Part model, mm, in its own coordinate system. Coordinates: 2 decimals unless noted, no trailing zeros. Order: outer loops, then holes, each group sorted by start corner. A loop starts at its lowest first (then second) coordinate and runs counter-clockwise, first axis right, second up. Notation, with made-up numbers: M -18.5,-19 L -5.5,-19 A34 cw -5.5,14 Z; hole C -39,53.5 d1. An arc over 180 degrees is marked long. Write item = value, one per line. Start each with the question number.
Autodesk Inventor part; units mm, degrees
ref_plane "YZ Plane" through (0, 0, 0) normal (1, 0, 0) x (0, 1, 0)
ref_plane "XZ Plane" through (0, 0, 0) normal (0, 1, 0) x (-1, 0, 0)
ref_plane "XY Plane" through (0, 0, 0) normal (0, 0, 1) x (1, 0, 0)
sketch "Sketch1" plane through (0, 0, 0) normal (0, 1, 0) x (-1, 0, 0)
  line L0 (0, 0) -> (53.34, 0)
  line L1 (53.34, 0) -> (53.34, -78.74)
  line L2 (53.34, -78.74) -> (0, -78.74)
  line L3 (0, -78.74) -> (0, 0)
  circle A0 centre (47.3075, -6.35) radius 2.54
  circle A1 centre (47.3075, -60.325) radius 2.54
  circle A2 centre (47.3075, -69.85) radius 2.54
  circle A3 centre (6.0325, -6.35) radius 2.54
  circle A4 centre (6.0325, -60.325) radius 2.54
  circle A5 centre (6.0325, -69.85) radius 2.54
  line L4 (26.67, 0) -> (26.67, -78.74)
  dimension "d0" = 53.34
  dimension "d1" = 78.74
  dimension "d2" = 5.08
  dimension "d3" = 5.08
  dimension "d4" = 5.08
  dimension "d5" = 53.975
  dimension "d6" = 63.5
  dimension "d9" = 41.275
  dimension "d14" = 20.6375
  dimension "d16" = 6.35
extrude "Extrusion1" add sketch "Sketch1" along normal blind 2.54
sketch "Sketch2" plane through (0, 2.54, 0) normal (0, 1, 0) x (1, 0, 0)
  line L0 (-53.34, 0) -> (0, 0)
  line L1 (-53.34, 78.74) -> (-53.34, 0)
  line L2 (0, 78.74) -> (-53.34, 78.74)
  line L3 (0, 0) -> (0, 78.74)
  circle A0 centre (-6.0325, 6.35) radius 2.54
  circle A1 centre (-6.0325, 60.325) radius 2.54
  circle A2 centre (-6.0325, 69.85) radius 2.54
  circle A3 centre (-47.3075, 69.85) radius 2.54
  circle A4 centre (-47.3075, 60.325) radius 2.54
  circle A5 centre (-47.3075, 6.35) radius 2.54
  line L4 (-26.67, 0) -> (-26.67, 78.74)
  line L5 (0, 78.74) -> (-53.34, 78.74)
  line L6 (-26.67, 0) -> (-39.37, 0)
  line L7 (-39.37, 0) -> (-39.37, 78.74)
  line L8 (-39.37, 78.74) -> (-26.67, 78.74)
  line L9 (-26.67, 78.74) -> (-26.67, 0)
  line L10 (-26.67, 0) -> (-13.97, 0)
  line L11 (-13.97, 0) -> (-13.97, 78.74)
  line L12 (-13.97, 78.74) -> (-26.67, 78.74)
  line L13 (-26.67, 78.74) -> (-26.67, 0)
  line L14 (-39.37, 0) -> (-40.386, 0)
  line L15 (-40.386, 0) -> (-40.386, 78.74)
  line L16 (-40.386, 78.74) -> (-39.37, 78.74)
  line L17 (-39.37, 78.74) -> (-39.37, 0)
  line L18 (-26.67, 0) -> (-27.178, 0)
  line L19 (-27.178, 0) -> (-27.178, 78.74)
  line L20 (-27.178, 78.74) -> (-26.67, 78.74)
  line L21 (-26.67, 78.74) -> (-26.67, 0)
  line L22 (-53.34, 0) -> (0, 0)
  line L23 (-26.67, 78.74) -> (-26.162, 78.74)
  line L24 (-26.162, 78.74) -> (-26.162, 0)
  line L25 (-26.162, 0) -> (-26.67, 0)
  line L26 (-26.67, 0) -> (-26.67, 78.74)
  line L27 (-13.97, 0) -> (-12.954, 0)
  line L28 (-12.954, 0) -> (-12.954, 78.74)
  line L29 (-12.954, 78.74) -> (-13.97, 78.74)
  line L30 (-13.97, 78.74) -> (-13.97, 0)
  line L31 (-40.386, 0) -> (-12.954, 0)
  line L32 (-12.954, 0) -> (-12.954, 1.27)
  line L33 (-12.954, 1.27) -> (-40.386, 1.27)
  line L34 (-40.386, 1.27) -> (-40.386, 0)
  line L35 (-12.954, 78.74) -> (-40.386, 78.74)
  line L36 (-40.386, 78.74) -> (-40.386, 77.47)
  line L37 (-40.386, 77.47) -> (-12.954, 77.47)
  line L38 (-12.954, 77.47) -> (-12.954, 78.74)
  line L39 (-53.34, 39.37) -> (0, 39.37)
  line L40 (0, 0) -> (0, 78.74)
  line L41 (-40.386, 39.37) -> (-12.954, 39.37)
  line L42 (-12.954, 39.37) -> (-12.954, 40.005)
  line L43 (-12.954, 40.005) -> (-40.386, 40.005)
  line L44 (-40.386, 40.005) -> (-40.386, 39.37)
  line L45 (-40.386, 39.37) -> (-12.954, 39.37)
  line L46 (-12.954, 39.37) -> (-12.954, 38.735)
  line L47 (-12.954, 38.735) -> (-40.386, 38.735)
  line L48 (-40.386, 38.735) -> (-40.386, 39.37)
  line L49 (-40.386, 38.735) -> (-39.37, 38.735)
  line L50 (-39.37, 38.735) -> (-39.37, 39.37)
  line L51 (-39.37, 39.37) -> (-40.386, 39.37)
  line L52 (-40.386, 39.37) -> (-40.386, 38.735)
  line L53 (-53.34, 78.74) -> (-53.34, 0)
  line L54 (-53.34, 0) -> (-52.324, 0)
  line L55 (-52.324, 0) -> (-52.324, 78.74)
  line L56 (-52.324, 78.74) -> (-53.34, 78.74)
  line L57 (-53.34, 78.74) -> (-53.34, 0)
  line L58 (0, 0) -> (-1.016, 0)
  line L59 (-1.016, 0) -> (-1.016, 78.74)
  line L60 (-1.016, 78.74) -> (0, 78.74)
  line L61 (0, 78.74) -> (0, 0)
  line L62 (-40.386, 39.37) -> (-53.34, 39.37)
  line L63 (-53.34, 39.37) -> (-53.34, 38.735)
  line L64 (-53.34, 38.735) -> (-40.386, 38.735)
  line L65 (-40.386, 38.735) -> (-40.386, 39.37)
  line L66 (-40.386, 39.37) -> (-53.34, 39.37)
  line L67 (-53.34, 39.37) -> (-53.34, 40.005)
  line L68 (-53.34, 40.005) -> (-40.386, 40.005)
  line L69 (-40.386, 40.005) -> (-40.386, 39.37)
  line L70 (-12.954, 39.37) -> (0, 39.37)
  line L71 (0, 39.37) -> (0, 38.735)
  line L72 (0, 38.735) -> (-12.954, 38.735)
  line L73 (-12.954, 38.735) -> (-12.954, 39.37)
  line L74 (-12.954, 39.37) -> (0, 39.37)
  line L75 (0, 39.37) -> (0, 40.005)
  line L76 (0, 40.005) -> (-12.954, 40.005)
  line L77 (-12.954, 40.005) -> (-12.954, 39.37)
  line L78 (-53.34, 38.735) -> (-52.324, 38.735)
  line L79 (-52.324, 38.735) -> (-52.324, 39.37)
  line L80 (-52.324, 39.37) -> (-53.34, 39.37)
  line L81 (-53.34, 39.37) -> (-53.34, 38.735)
  point P0 (-13.97, 38.735)
  point P1 (-13.97, 40.005)
  point P2 (-27.178, 38.735)
  point P3 (-26.162, 38.735)
  point P4 (-26.162, 40.005)
  point P5 (-27.178, 40.005)
  point P6 (-13.97, 1.27)
  point P7 (-27.178, 1.27)
  point P8 (-26.162, 1.27)
  point P9 (-39.37, 1.27)
  point P10 (-13.97, 77.47)
  point P11 (-27.178, 77.47)
  point P12 (-26.162, 77.47)
  point P13 (-39.37, 77.47)
  point P14 (-39.37, 38.735)
  point P15 (-39.37, 40.005)
  point P16 (-1.016, 38.735)
  point P17 (-1.016, 40.005)
  point P18 (-52.324, 38.735)
  point P19 (-52.324, 40.005)
  dimension "d19" = 12.7
  dimension "d20" = 12.7
  dimension "d22" = 0.508
  dimension "d23" = 0.508
  dimension "d24" = 1.016
  dimension "d25" = 1.016
  dimension "d26" = 1.27
  dimension "d27" = 1.27
  dimension "d28" = 0.635
  dimension "d29" = 0.635
  dimension "d32" = 1.016
  dimension "d33" = 1.016
extrude "Extrusion3" add sketch "Sketch2" along normal blind 0.5 contours L1 L39 L55 L64 | L15 L33 L7 L0 | L1 L68 L55 L39 | L19 L33 L4 L0 | L4 L33 L24 L0 | L15 L2 L7 L37 | L11 L33 L28 L0 | L19 L2 L4 L37 | L4 L2 L24 L37 | L59 L39 L3 L72 | L59 L76 L3 L39 | L11 L2 L28 L37
properties part number "trucks"
Item 1: Cut at C-C, the plane z = -10. Write the cut outline in (x, y), and give its area (3 significant figures).
Item 2: Cut at B-B, the plane y = 1.35. Count the separate pieces of the cut face and the enclosed holes in it, and give its area (3 significant figures).
Item 3: Cut at A-A, the plane z = -69.85. Write the cut outline in (x, y).
Item 4: Wall check: line 1 along X through (y, z) = (1.3, -60.5); line 2 along Z through (x, y) = (-5, 1.95); line 3 along Y through (x, z) = (-13, -37). Give the ranges that are in metal, low to high. Write a range as [from, to].
Item 5: Flat gauge pins, fed straight in: pin 1 (0.6 mm diameter, centred on y = 3, z = -0.5, fed in from -X); pin 2 (0.6 mm diameter, centred on y = 3, z = -78, fed in from +X); pin 3 (1.5 mm diameter, centred on x = -28, z = -47.5, fed in from +Y). Where does each tip first touch, or does it go through?
Item 6: Pull direction X, two halves, no side cores. Call faces 1 (the flat face through (-26, 1, 0)), 2 (the flat face through (-53.34, 1, -39)), 3 (the cylindrical face through (-5.48, 1.25, -67.37)): pulls with the +X half, pulls with the -X half, needs draft (parallel to the pull), parting line crosses it, or undercut.
Filled sheet:
q1.outline = M -53.34,0 L 0,0 L 0,2.54 L -53.34,2.54 Z
q1.area = 135 mm2
q2.separate_pieces = 1
q2.enclosed_holes = 6
q2.area = 4,080 mm2
q3.outline = M -53.34,0 L -49.85,0 L -49.85,2.54 L -53.34,2.54 Z; M -44.77,0 L -8.57,0 L -8.57,2.54 L -44.77,2.54 Z; M -3.49,0 L 0,0 L 0,2.54 L -3.49,2.54 Z
q4.line_1 = [-53.34, -49.84], [-44.77, -8.57], [-3.5, 0]
q4.line_2 = [-78.74, -72.17], [-67.53, -62.65], [-58, -8.67], [-4.03, 0]
q4.line_3 = [0, 2.54]
q5.pin_1 = -40.39
q5.pin_2 = -12.95
q5.pin_3 = 2.54
q6.face_1 = needs draft
q6.face_2 = pulls with the -X half
q6.face_3 = undercut
